The listing builds one solid part. Answer for the finished solid, in the listing's coordinates (mm). Round coordinates to 2 decimals unless told otherwise and drop trailing zeros. Write each loop counter-clockwise with the first axis right and the second up, starting at its lowest first coordinate (ties: lowest second). Pieces come first, ordered by that corner, then holes. Notation, with made-up numbers: M -15.75,58 L 16.25,58 A14 ccw 16.25,77 Z; hole C 33,41 d5. An arc over 180 degrees is marked long. Write each question's results on one line, items separated by ' | '.
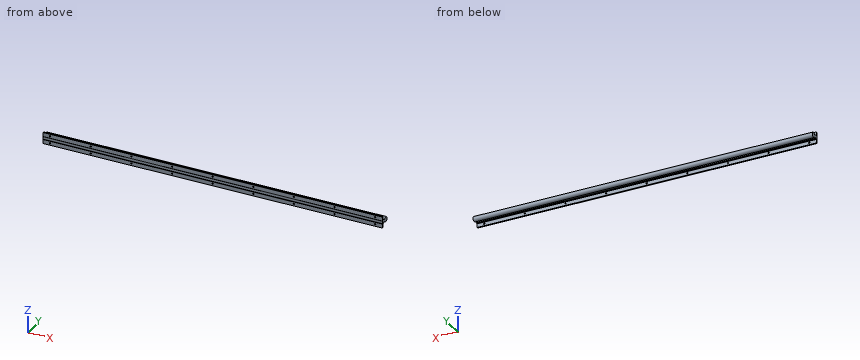
from build123d import *

# Parameters (mm, degrees)
EXTRUDE_1_DEPTH         = 1670
HOLE_WIZARD_6_6_6_6_1_D = 6.6
PATTERN_LINEAR_1_COUNT  = 9
PATTERN_LINEAR_1_PITCH  = 200


with BuildPart() as part:
    # 草图1 → 凸台-拉伸1 (new body)
    with BuildSketch(Plane(origin=(0, 0, 0), x_dir=(0, 0, -1), z_dir=(1, 0, 0))):
        with BuildLine():
            Line((38.023703704, 12.710240583), (38.023703704, 6.710240583))
            Line((38.023703704, 6.710240583), (18.023703704, 6.710240583))
            Line((18.023703704, 6.710240583), (16.823703704, 7.910240583))
            Line((16.823703704, 7.910240583), (4.223703704, 7.910240583))
            Line((4.223703704, 7.910240583), (3.023703704, 6.710240583))
            Line((3.023703704, 6.710240583), (-16.976296296, 6.710240583))
            Line((-16.976296296, 6.710240583), (-16.976296296, 12.710240583))
            Line((-16.976296296, 12.710240583), (1.023703704, 12.710240583))
            Line((1.023703704, 12.710240583), (1.023703704, 19.410240583))
            Line((1.023703704, 19.410240583), (2.593703704, 19.410240583))
            Line((2.593703704, 19.410240583), (5.975416608, 28.06708446))
            ThreePointArc((5.975416608, 28.06708446), (10.523703704, 52.210240583), (15.0719908, 28.06708446))
            Line((15.0719908, 28.06708446), (18.453703704, 19.410240583))
            Line((18.453703704, 19.410240583), (20.023703704, 19.410240583))
            Line((20.023703704, 19.410240583), (20.023703704, 12.710240583))
            Line((20.023703704, 12.710240583), (38.023703704, 12.710240583))
        make_face()
    extrude(amount=EXTRUDE_1_DEPTH)

    # Ø6.6 (6.6) 直径孔1 (through all)
    with Locations(Plane(origin=(35, 12.710240583, -28.023703704), x_dir=(0, 0, 1), z_dir=(0, 1, 0))):
        with Locations((0, 0), (35, 0)):
            hole_wizard_6_6_6_6_1 = Hole(HOLE_WIZARD_6_6_6_6_1_D / 2)

    # 阵列(线性)1: Ø6.6 (6.6) 直径孔1 ×9
    with Locations(*[(i * PATTERN_LINEAR_1_PITCH, 0, 0) for i in range(1, PATTERN_LINEAR_1_COUNT)]):
        add(hole_wizard_6_6_6_6_1, mode=Mode.SUBTRACT)


solid = part.part
1) Section B-B (y = 44) is taken. Determine the outline of the cut face in (x, z), then the cut area to 3 significant figures.
Return value:
outline: M 0,-22.26 L 1670,-22.26 L 1670,1.22 L 0,1.22 Z | area: 39,200 mm²
2) Each of these flat-tipped pins is pushed along its axis until it touches: pin 1 (6 mm diameter, centred on x = 1068.5, y = 36, fed in from -Z); pin 2 (1.5 mm diameter, centred on x = 439, y = 19, fed in from -Z); pin 3 (1 mm diameter, centred on x = 174, z = -21, fed in from +Y); pin 4 (8 mm diameter, centred on x = 727.5, z = -9.5, fed in from +Y). Where does it stop, or does it pass through?
Return value:
pin 1: z = -23 | pin 2: z = -20.02 | pin 3: y = 47.24 | pin 4: y = 52.21
3) Find the intervals of material crossed by line 1 (Z direction, x = 1635, y = 10); line 2 (Z direction, x = 1548, y = 29); line 3 (Y direction, x = 1186, z = -32.5), in increasing order.
Return value:
line 1: -38.02 to -31.32, -24.72 to 3.68, 10.28 to 16.98 | line 2: -16.97 to -4.08 | line 3: 6.71 to 12.71
4) Section A-A (x = 1566) is taken. Determine the outline of the cut face in (y, z).
Return value:
outline: M 6.71,-38.02 L 12.71,-38.02 L 12.71,-20.02 L 19.41,-20.02 L 19.41,-18.45 L 28.07,-15.07 A12.5 ccw long 28.07,-5.98 L 19.41,-2.59 L 19.41,-1.02 L 12.71,-1.02 L 12.71,16.98 L 6.71,16.98 L 6.71,-3.02 L 7.91,-4.22 L 7.91,-16.82 L 6.71,-18.02 Z
